from build123d import *

# Parameters (mm, degrees)
EXTRUDE_1_DEPTH = 4.8
SKETCH_2_R      = 3
EXTRUDE_2_DEPTH = 4
FILLET_4_R      = 0.7
CHAMFER_1_SIZE  = 0.4


with BuildPart() as part:
    # Эскиз1 → Бобышка-Вытянуть1 (new body)
    with BuildSketch(Plane(origin=(0, 0, 0), x_dir=(1, 0, 0), z_dir=(0, 1, 0))):
        Polygon((4.041451884, 0), (2.020725942, 3.5), (-2.020725942, 3.5), (-4.041451884, 0), (-2.020725942, -3.5), (2.020725942, -3.5), align=None)
    extrude(amount=EXTRUDE_1_DEPTH)

    # Эскиз2 → Бобышка-Вытянуть2 (add)
    with BuildSketch(Plane(origin=(0, 4.8, 0), x_dir=(1, 0, 0), z_dir=(0, 1, 0))):
        with Locations(Location((0, 0, 0), (0, 0, 270))):
            Circle(SKETCH_2_R)
    extrude(amount=EXTRUDE_2_DEPTH)

    # Скругление4
    fillet_4_edges = [part.edges().sort_by_distance(p)[0] for p in [
        (0, 4.8, -3),
    ]]
    fillet(fillet_4_edges, radius=FILLET_4_R)

    # Фаска1
    chamfer_1_edges = [part.edges().sort_by_distance(p)[0] for p in [
        (0, 8.8, -3),
    ]]
    chamfer(chamfer_1_edges, length=CHAMFER_1_SIZE)


solid = part.part
Verification items for the finished model (mm, model axes). A direction names the side the tool comes from. Give positions to 0.01 mm unless a question says otherwise; leave off trailing zeros. Order: outer loops, then holes, each group sorted by start corner. A loop starts at its lowest first (then second) coordinate and runs counter-clockwise, first axis right, second up. Notation, with made-up numbers: (50.25, 40.25) -> (109.25, 40.25) arc R14 ccw to (109.25, 59.25) -> close; hole circle Ø3 at (42, 9.25). An arc over 180 degrees is marked (long way). Answer as CSV lines item,"result".
Q1. Access from +Z, -Z, +X, -X, +Y, -Y to the whole of each face (thin tool, end or side, straight path). Record for faces 1 (the flat face through (0, 0, 0)), 2 (the cylindrical face through (-1.15, 6.91, 2.77)).
Solutions:
face 1,"+Z, -Z, +X, -X, -Y"
face 2,"+Y"
Q2. Scan lines: probe 1 along X at (y, z) = (3.5, 2.5); probe 2 along X at (y, z) = (6.75, 2.75). Record each from-to range of solid material in increasing order.
Solutions:
probe 1,"x = -2.6 to 2.6"
probe 2,"x = -1.2 to 1.2"
Q3. Depth check by flat-ended pin: pin 1 (2 mm diameter, centred on x = -2.5, z = 1.5, fed in from -Y); pin 2 (1.5 mm diameter, centred on x = -1.5, y = 7, fed in from +Z); pin 3 (0.8 mm diameter, centred on x = -2, z = 3, fed in from +Y); pin 4 (3 mm diameter, centred on y = 1.5, z = 3, fed in from +X). Enter the tip coordinate at first touch or a pass-through.
Solutions:
pin 1,"stops at y = 0"
pin 2,"stops at z = 2.9"
pin 3,"stops at y = 5"
pin 4,"stops at x = 3.18"
Q4. Sectioned sample at A-A on y = 3. Record the cut outline in (x, z), plus the area to 3 significant figures.
Solutions:
outline,"(-4.04, 0) -> (-2.02, -3.5) -> (2.02, -3.5) -> (4.04, 0) -> (2.02, 3.5) -> (-2.02, 3.5) -> close"
area,"42.4 mm²"
Q5. Sectioned sample at B-B on y = 6. Record the cut outline in (x, z), plus the area to 3 significant figures.
Solutions:
outline,"circle Ø6 at (0, 0)"
area,"28.3 mm²"
